from build123d import *

# Parameters (mm, degrees)
F1_DEPTH = 48
F2_DEPTH = 2
F3_R     = 0.5


with BuildPart() as f1:
    # F0 (on Top) → F1 (new body)
    with BuildSketch(Plane.XY):
        with BuildLine():
            Line((0, 2.75), (0, 5))
            ThreePointArc((0, 5), (-5, 0), (0, -5))
            Line((0, -5), (0, -2.75))
            ThreePointArc((0, -2.75), (-2.75, 0), (0, 2.75))
        make_face()
    extrude(amount=F1_DEPTH)

    # F0 (on Top) → F2 (join)
    with BuildSketch(Plane.XY):
        with BuildLine():
            Line((0, 2.75), (0, 5))
            ThreePointArc((0, 5), (-5, 0), (0, -5))
            Line((0, -5), (0, -2.75))
            ThreePointArc((0, -2.75), (-2.75, 0), (0, 2.75))
        make_face()
        with BuildLine():
            Line((0, -2.75), (0, 2.75))
            ThreePointArc((0, 2.75), (-2.75, 0), (0, -2.75))
        make_face()
    extrude(amount=F2_DEPTH)

    # F3
    f3_edges = [f1.edges().sort_by_distance(p)[0] for p in [
        (0, 2.75, 25),
        (0, -2.75, 25),
        (0, -5, 24),
        (0, 0, 2),
        (0, 5, 24),
    ]]
    fillet(f3_edges, radius=F3_R)


solid = f1.part
Work out the finished part from the listing and answer in its coordinate system (mm). A direction names the side the tool comes from. Coordinates: 2 decimals unless noted, no trailing zeros. Write each loop counter-clockwise with the first axis right and the second up, starting at its lowest first coordinate (ties: lowest second). Pieces come first, ordered by that corner, then holes.
1. The part is cut by section C-C, the plane x = -1.55. Write down the section's boundary in (y, z), and give its area (3 significant figures).
Results list:
outline: (-4.75, 0) - (4.75, 0) - (4.75, 48) - (2.27, 48) - (2.27, 2) - (-2.27, 2) - (-2.27, 48) - (-4.75, 48) - close
area: 247 mm2
2. For a pull along Y with two mould halves and no side action, classify faces 3 (the cylindrical face through (-5, 0, 24)), 4 (the flat face through (-1, 0, 2)), 5 (the flat face through (0, -4, 22)) as +Y half, -Y half, draft (parallel to the pull), parting line (faces both ways), or undercut.
Results list:
face 3: parting line
face 4: undercut
face 5: draft
3. A flat-ended cylindrical pin translates along its axis: pin 1 (2 mm diameter, centred on x = -2.5, z = 38.5, fed in from -Y). Find the tip coordinate at first contact, or state that the pin passes through.
Results list:
pin 1: stops at y = -4.77
4. The part is cut by section D-D, the plane y = 4. Write down the section's boundary in (x, z), and give its area (3 significant figures).
Results list:
outline: (-3, 0) - (0, 0) - (0, 48) - (-3, 48) - close
area: 144 mm2
5. Consider line 1 along Y through (x, z) = (-1.85, 42); line 2 along Y through (x, z) = (-2.25, 21); line 3 along X through (y, z) = (0.5, 34). Determine where each line is inside the solid, lowest interval first.
Results list:
line 1: y = -4.65 to -2.03, 2.03 to 4.65
line 2: y = -4.47 to -1.58, 1.58 to 4.47
line 3: x = -4.97 to -2.7
6. The part is cut by section B-B, the plane y = -2. Write down the section's boundary in (x, z).
Results list:
outline: (-4.58, 0) - (0, 0) - (0, 1.5) arc R0.5 ccw to (-0.5, 2) - (-1.89, 2) - (-1.89, 48) - (-4.58, 48) - close
7. For faces 1 (the flat face through (-3, 0, 48)), 2 (the cylindrical face through (-2.75, -0.05, 24.67)), determine the directions among +Z, -Z, +X, -X, +Y, -Y from which every point of the face is accessible in a straight line to the end or side of a thin tool.
Results list:
face 1: +Z, +X, -X, +Y, -Y
face 2: +Z, +X
8. The part is cut by section A-A, the plane z = 19.5. Write down the section's boundary in (x, y), and give its area (3 significant figures).
Results list:
outline: (-0.56, -4.97) arc R0.5 ccw to (0, -4.47) - (0, -3.21) arc R0.5 ccw to (-0.42, -2.72) arc R2.75 cw to (-0.42, 2.72) arc R0.5 ccw to (0, 3.21) - (0, 4.47) arc R0.5 ccw to (-0.56, 4.97) arc R5 ccw to start
area: 27.2 mm2
